Can you work these out from the model? Positions are in its coordinate system, mm. A direction names the side the tool comes from. Coordinates: 2 decimals unless noted, no trailing zeros. Order: outer loops, then holes, each group sorted by start corner. A loop starts at its lowest first (then second) coordinate and runs counter-clockwise, first axis right, second up. Notation, with made-up numbers: (72.5, -16.5) -> (82.5, -16.5) arc R19 cw to (82.5, -7.5) -> close; hole circle Ø10 at (7.5, -38). An arc over 180 degrees is marked (long way). Use a Markdown table: item, result. Add a question column.
1. Suppose I cut it at C-C, the plane z = 10. List the corners of the cut face in (x, y) for me, then the cut area to 3 significant figures.
2. For pin 1 Ø2 at (x, z) = (-34, 13.5) entering from -Y; pin 2 Ø12 at (y, z) = (29.5, 23) entering from +X; pin 3 Ø4 at (x, y) = (-15, 16) entering from -Z; pin 4 Ø7.5 at (y, z) = (36.5, 38.5) entering from +X, each with a flat end and sliding along its axis, tell me the tip position at first contact or that it passes through.
3. For faces 4 (the flat face through (-45, 45, 25)), 5 (the flat face through (0, 45, 44)), 6 (the flat face through (-25, 24, 2)), 7 (the cylindrical face through (3, 10, 45)), 8 (the flat face through (0, 5, 45)), which set-ups out of +Z, -Z, +X, -X, +Y, -Y let a thin tool reach every point of the face, with its end or its side?
4. If I drill on line 1 along Z through (x, y) = (-3, 39.5); line 2 along Y through (x, z) = (-15, 49), over which ranges is the centre line in solid material (lowest first)? Write a range as from..to.
5. Suppose I cut it at B-B, the plane x = -15. List the corners of the cut face in (y, z) for me.
6. We'd pull the mould along X, two halves only. Please class faces 1 (the flat face through (-50, 25, 25)), 2 (the flat face through (-21, 48, 25)), 3 (the flat face through (0, 45, 6)): pulls with the +X half, pulls with the -X half, needs draft (parallel to the pull), parting line crosses it, or undercut.
7. Suppose I cut it at D-D, the plane y = 6. List the corners of the cut face in (x, z) for me.
8. Suppose I cut it at A-A, the plane y = 17. List the corners of the cut face in (x, z) for me.
```python
from build123d import *

# Parameters (mm, degrees)
BOSS_EXTRU_1_DEPTH      = 50
ESQUISSE3_R             = 25
BOSS_EXTRU_2_DEPTH      = 7
ESQUISSE4_R             = 2.5
ENL_V_MAT_EXTRU_1_DEPTH = 87.602540378
COQUE1_START            = -39.171572875
COQUE1_OUTLINE_W        = 48
COQUE1_OUTLINE_H        = 46
COQUE1_DEPTH            = 37.171572875
COQUE1_START_2          = -2
COQUE1_2_OUTLINE_R      = 23
COQUE1_2_DEPTH          = 9
COQUE1_START_3          = -48
COQUE1_3_DEPTH          = 15.9452
COQUE1_START_4          = 2
COQUE1_4_DEPTH          = 46


with BuildPart() as part:
    # Esquisse1 → Boss.-Extru.1 (new body)
    with BuildSketch(Plane.XY):
        Polygon((0, 0), (-30, 0), (-50, 10), (-50, 40), (-40, 50), (0, 50), align=None)
    extrude(amount=BOSS_EXTRU_1_DEPTH)

    # Esquisse3 → Boss.-Extru.2 (add)
    with BuildSketch(Plane(origin=(0, 0, 0), x_dir=(0, 0, -1), z_dir=(1, 0, 0))):
        with Locations((-25, 25)):
            Circle(ESQUISSE3_R)
    extrude(amount=BOSS_EXTRU_2_DEPTH)

    # Esquisse4 → Enlèv. mat.-Extru.1 (cut, through all)
    with BuildSketch(Plane.XY.offset(50)):
        with Locations((-15, 16)):
            Circle(ESQUISSE4_R)
    extrude(amount=-ENL_V_MAT_EXTRU_1_DEPTH, mode=Mode.SUBTRACT)

    # Coque1: read off the stored shape, not the designer's step
    # Coque1 outline → Coque1 (cut)
    with BuildSketch(Plane.YZ.offset(COQUE1_START)):
        with Locations((24, 25)):
            Rectangle(COQUE1_OUTLINE_W, COQUE1_OUTLINE_H)
    extrude(amount=COQUE1_DEPTH, mode=Mode.SUBTRACT)

    # Coque1 2 outline → Coque1 2 (cut)
    with BuildSketch(Plane.YZ.offset(COQUE1_START_2)):
        with Locations((25, 25)):
            Circle(COQUE1_2_OUTLINE_R)
    extrude(amount=COQUE1_2_DEPTH, mode=Mode.SUBTRACT)

    # Coque1 3 outline → Coque1 3 (cut)
    with BuildSketch(Plane.YZ.offset(COQUE1_START_3)):
        with BuildLine():
            ThreePointArc((25, 2), (2, 25), (25, 48))
            Line((25, 48), (0, 48))
            Line((0, 48), (0, 2))
            Line((0, 2), (25, 2))
        make_face()
    extrude(amount=COQUE1_3_DEPTH, mode=Mode.SUBTRACT)

    # Coque1 4 outline → Coque1 4 (cut)
    with BuildSketch(Plane.XY.offset(COQUE1_START_4)):
        Polygon((-39.171572875, 48), (-48, 39.171572875), (-48, 9), (-39.171572875, 4.585786437), align=None)
    extrude(amount=COQUE1_4_DEPTH, mode=Mode.SUBTRACT)


solid = part.part
```
Worked out:
| question | item | result |
|---|---|---|
| 1 | outline | (-50, 10) -> (-48, 9) -> (-48, 39.17) -> (-39.17, 48) -> (-2, 48) -> (-2, 42.44) -> (7, 42.44) -> (7, 45) -> (0, 45) -> (0, 50) -> (-40, 50) -> (-50, 40) -> close; (-2, 0) -> (0, 0) -> (0, 5) -> (7, 5) -> (7, 7.56) -> (-2, 7.56) -> close |
| 1 | area | 228 mm² |
| 2 | pin 1 | stops at y = 48 |
| 2 | pin 2 | stops at x = -48 |
| 2 | pin 3 | passes through |
| 2 | pin 4 | stops at x = -46.92 |
| 3 | face 4 | +Z, -Z, -X, +Y |
| 3 | face 5 | +Z, +X, +Y |
| 3 | face 6 | -Y |
| 3 | face 7 | +X |
| 3 | face 8 | +Z, +X, -Y |
| 4 | line 1 | z = 0..2, 48..50 |
| 4 | line 2 | y = 0..13.5, 18.5..50 |
| 5 | outline | (0, 0) -> (13.5, 0) -> (13.5, 2) -> (0, 2) -> close; (0, 48) -> (13.5, 48) -> (13.5, 50) -> (0, 50) -> close; (18.5, 0) -> (50, 0) -> (50, 50) -> (18.5, 50) -> (18.5, 48) -> (48, 48) -> (48, 2) -> (18.5, 2) -> close |
| 6 | face 1 | pulls with the -X half |
| 6 | face 2 | undercut |
| 6 | face 3 | pulls with the +X half |
| 7 | outline | (-42, 0) -> (0, 0) -> (0, 8.75) -> (7, 8.75) -> (7, 12.04) -> (-2, 12.04) -> (-2, 2) -> (-42, 2) -> close; (-42, 48) -> (-2, 48) -> (-2, 37.96) -> (7, 37.96) -> (7, 41.25) -> (0, 41.25) -> (0, 50) -> (-42, 50) -> close |
| 8 | outline | (-50, 0) -> (-17.29, 0) -> (-17.29, 2) -> (-48, 2) -> (-48, 48) -> (-17.29, 48) -> (-17.29, 50) -> (-50, 50) -> close; (-12.71, 0) -> (0, 0) -> (0, 1.31) -> (7, 1.31) -> (7, 3.44) -> (-2, 3.44) -> (-2, 2) -> (-12.71, 2) -> close; (-12.71, 48) -> (-2, 48) -> (-2, 46.56) -> (7, 46.56) -> (7, 48.69) -> (0, 48.69) -> (0, 50) -> (-12.71, 50) -> close |
